from build123d import *

# Parameters (mm, degrees)
F0_W     = 152.4
F0_H     = 76.2
F1_DEPTH = 25.4
F2_W     = 39.9509807944
F2_H     = 76.2
F3_DEPTH = 50.8
F4_W     = 36.2490192056
F4_H     = 20.8374331653
F4_H_2   = 18.6278219283
F5_DEPTH = 25.4


with BuildPart() as f1:
    # F0 (on Top) → F1 (new body)
    with BuildSketch(Plane.XY):
        Rectangle(F0_W, F0_H)
    extrude(amount=F1_DEPTH)

    # F2 (on face) → F3 (join)
    with BuildSketch(Plane.XY.offset(25.4)):
        with Locations((-56.2245096028, 0)):
            Rectangle(F2_W, F2_H)
    extrude(amount=F3_DEPTH)

    # F4 (on face) → F5 (join)
    with BuildSketch(Plane.XY.offset(25.4)):
        with Locations((-18.1245096028, 27.6812834173)):
            Rectangle(F4_W, F4_H)
        with Locations((-18.1245096028, -28.7860890359)):
            Rectangle(F4_W, F4_H_2)
    extrude(amount=F5_DEPTH)


solid = f1.part
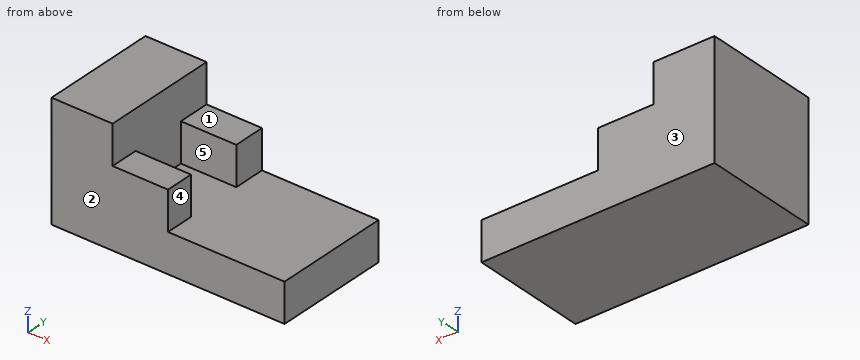
Design review of the part built by this model. Coordinates are the model's own, in mm. Face numbers are marked on the shaded views. A direction names the side the tool comes from. Round coordinates to 2 decimals unless told otherwise and drop trailing zeros. Loops run counter-clockwise (first coordinate to the right, second up) from the corner with the lowest first, then second, coordinate; pieces in that order, holes last. Notation, with made-up numbers: (22.25, 9.25) - (54.25, 9.25) arc R26 ccw to (54.25, 28.25) - close; hole circle Ø3 at (7.25, 58.25). An arc over 180 degrees is marked (long way). One line per item, written item: value. Start each with the question number.
1) Consider section A-A on y = -28. Give the boundary of the cut face in (x, z), then the cut area to 3 significant figures.
2) For the marked faces 1 and 2, list the 3-axis set-ups (+Z, -Z, +X, -X, +Y, -Y) from which the entire face can be reached by the end or side of a thin tool; tool diameter is ignored.
3) Consider section C-C on z = 65. Give the boundary of the cut face in (x, y).
4) Consider section D-D on y = 15.5. Give the boundary of the cut face in (x, z), then the cut area to 3 significant figures.
5) Insertion check: pin 1 Ø16.5 at (y, z) = (30, 38) entering from +X; pin 2 Ø9.5 at (x, y) = (-13.5, -25) entering from +Z; pin 3 Ø10 at (x, y) = (35, 3.5) entering from +Z. Each pin has a flat end and moves straight along its axis. Give the tip position at first contact, or say it passes through.
6) Consider section B-B on x = -34. Give the boundary of the cut face in (y, z).
7) To check wall thickness, follow L1, parallel to Y at x = -32, z = 34; L2, parallel to X at y = -21.5, z = 54.5; L3, parallel to Z at x = 6, y = 25. State the ranges of each line that lie inside material, in increasing order. Write a range as from..to.
8) Draft analysis for pull direction Y (two halves, no side actions). For the marked faces 3, 4 and 5, state which applies: +Y half, -Y half, draft (parallel to the pull), parting line (faces both ways), or undercut.
Reported:
1. outline: (-76.2, 0) - (76.2, 0) - (76.2, 25.4) - (0, 25.4) - (0, 50.8) - (-36.25, 50.8) - (-36.25, 76.2) - (-76.2, 76.2) - close
1. area: 6,820 mm^2
2. face 1: +Z, +X, +Y, -Y
2. face 2: +Z, -Z, +X, -X, -Y
3. outline: (-76.2, -38.1) - (-36.25, -38.1) - (-36.25, 38.1) - (-76.2, 38.1) - close
4. outline: (-76.2, 0) - (76.2, 0) - (76.2, 25.4) - (-36.25, 25.4) - (-36.25, 76.2) - (-76.2, 76.2) - close
4. area: 5,900 mm^2
5. pin 1: stops at x = 0
5. pin 2: stops at z = 50.8
5. pin 3: stops at z = 25.4
6. outline: (-38.1, 0) - (38.1, 0) - (38.1, 50.8) - (17.26, 50.8) - (17.26, 25.4) - (-19.47, 25.4) - (-19.47, 50.8) - (-38.1, 50.8) - close
7. L1: y = -38.1..-19.47, 17.26..38.1
7. L2: x = -76.2..-36.25
7. L3: z = 0..25.4
8. face 3: +Y half
8. face 4: draft
8. face 5: undercut
